Can you work these out from the model? Positions are in its coordinate system, mm. Face numbers are marked on the shaded views. A direction names the side the tool comes from. Give positions to 0.01 mm unless a question says otherwise; leave off trailing zeros. Loops run counter-clockwise (first coordinate to the right, second up) from the corner with the lowest first, then second, coordinate; pieces in that order, holes last. Notation, with made-up numbers: M -33.75,-26 L -3.75,-26 A36 cw -3.75,13 Z; hole C -21.75,53.25 d11. An arc over 180 degrees is marked long. Answer as a JSON object with one key per item and string values.
```python
from build123d import *

# Parameters (mm, degrees)
BOSS_EXTRUDE1_DEPTH = 25.4
SKETCH2_R           = 6.35
BOSS_EXTRUDE2_DEPTH = 101.6


with BuildPart() as part:
    # Sketch1 → Boss-Extrude1 (new body)
    with BuildSketch(Plane.XY):
        Polygon((0, 0), (97.980047506, 0), (97.980047506, 101.6), (0, 101.6), (0, 114.3), (110.680047506, 114.3), (110.680047506, -12.7), (0, -12.7), align=None)
    extrude(amount=BOSS_EXTRUDE1_DEPTH)

    # Sketch2 → Boss-Extrude2 (add)
    with BuildSketch(Plane(origin=(0, 0, 0), x_dir=(1, 0, 0), z_dir=(0, 1, 0))):
        with Locations(Location((40.640027753, -12.7, 0), (0, 0, 90))):
            Circle(SKETCH2_R)
        with Locations(Location((57.340019753, -12.7, 0), (0, 0, 90))):
            Circle(SKETCH2_R)
    extrude(amount=BOSS_EXTRUDE2_DEPTH)


solid = part.part
```
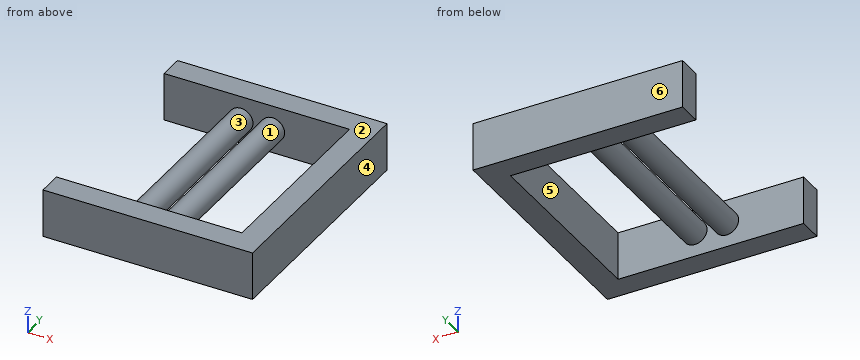
1) Suppose I cut it at B-B, the plane z = 12.7. Write out the boundary of the cut face in (x, y).
Answer list:
{"outline": "M 0,-12.7 L 110.68,-12.7 L 110.68,114.3 L 0,114.3 L 0,101.6 L 34.29,101.6 L 34.29,0 L 0,0 Z; hole M 46.99,0 L 50.99,0 L 50.99,101.6 L 46.99,101.6 Z; hole M 63.69,0 L 97.98,0 L 97.98,101.6 L 63.69,101.6 Z"}
2) Please list where these lines run through material, in increasing order: line 1 along X through (y, z) = (40, 12.25); line 2 along Y through (x, z) = (28, 2); line 3 along X through (y, z) = (97, 18.5). Write a range as from..to.
Answer list:
{"line 1": "34.31..46.97, 51.01..63.67, 97.98..110.68", "line 2": "-12.7..0, 101.6..114.3", "line 3": "38.05..43.23, 54.75..59.93, 97.98..110.68"}
3) Suppose I cut it at D-D, the plane y = 28. Write out the boundary of the cut face in (x, z), and give its area (3 significant figures).
Answer list:
{"outline": "C 40.64,12.7 d12.7; C 57.34,12.7 d12.7; M 97.98,0 L 110.68,0 L 110.68,25.4 L 97.98,25.4 Z", "area": "576 mm^2"}
4) Will these pins go through, and if not, where does the flat tip stop? pin 1 Ø8 at (x, y) = (57, 93.5) entering from -Z; pin 2 Ø6 at (y, z) = (13.5, 22.5) entering from -X.
Answer list:
{"pin 1": "z = 6.35", "pin 2": "x = 97.98"}
5) Suppose I cut it at A-A, the plane x = 69.5. Write out the boundary of the cut face in (y, z), and give its area (3 significant figures).
Answer list:
{"outline": "M -12.7,0 L 0,0 L 0,25.4 L -12.7,25.4 Z; M 101.6,0 L 114.3,0 L 114.3,25.4 L 101.6,25.4 Z", "area": "645 mm^2"}
6) For the marked faces 1 and 2, which set-ups out of +Z, -Z, +X, -X, +Y, -Y let a thin tool reach every point of the face, with its end or its side?
Answer list:
{"face 1": "none", "face 2": "+Z, +X, -X, +Y, -Y"}
7) If we mould it in two halves opening along Y, with no side actions, what happens to the marked faces 3, 4, 5 and 6? For each: +Y half, -Y half, draft (parallel to the pull), parting line (faces both ways), or undercut.
Answer list:
{"face 3": "undercut", "face 4": "draft", "face 5": "undercut", "face 6": "+Y half"}
8) Suppose I cut it at C-C, the plane z = 2.75. Write out the boundary of the cut face in (x, y), and give its area (3 significant figures).
Answer list:
{"outline": "M 0,-12.7 L 110.68,-12.7 L 110.68,114.3 L 0,114.3 L 0,101.6 L 97.98,101.6 L 97.98,0 L 0,0 Z", "area": "4,100 mm^2"}
